```python
from build123d import *

# Parameters (mm, degrees)
F0_R     = 1.25
F1_DEPTH = 7


with BuildPart() as f1:
    # F0 (on Front) → F1 (new body)
    with BuildSketch(Plane.XZ):
        with BuildLine():
            Line((0, 7), (0, 0))
            Line((0, 0), (11, 0))
            Line((11, 0), (11, 7))
            Line((11, 7), (21, 7))
            Line((21, 7), (21, 12))
            Line((21, 12), (20, 12))
            Line((20, 12), (20, 15))
            Line((20, 15), (21, 15))
            Line((21, 15), (21, 21))
            Line((21, 21), (24, 21))
            Line((24, 21), (24, 15))
            Line((24, 15), (25, 15))
            Line((25, 15), (25, 12))
            Line((25, 12), (24, 12))
            Line((24, 12), (24, 7))
            Line((24, 7), (30, 7))
            Line((30, 7), (30, 26))
            Line((30, 26), (0, 26))
            Line((0, 26), (0, 20.75))
            ThreePointArc((0, 20.75), (0.368034, 20.309017), (0.5, 19.75))
            ThreePointArc((0.5, 19.75), (0.368034, 19.190983), (0, 18.75))
            Line((0, 18.75), (0, 7))
        make_face()
        with Locations((8.75, 19.75)):
            Circle(F0_R, mode=Mode.SUBTRACT)
        with BuildLine():
            Line((-5, 7), (0, 7))
            Line((0, 7), (0, 18.75))
            ThreePointArc((0, 18.75), (-2, 19.75), (0, 20.75))
            Line((0, 20.75), (0, 26))
            Line((0, 26), (-5, 26))
            Line((-5, 26), (-5, 7))
        make_face()
    extrude(amount=F1_DEPTH)


solid = f1.part
```
Input: part model. Units: mm. Frame: model coordinates. A direction names the side the tool comes from. Give positions to 0.01 mm unless a question says otherwise; leave off trailing zeros. Order: outer loops, then holes, each group sorted by start corner. A loop starts at its lowest first (then second) coordinate and runs counter-clockwise, first axis right, second up. Notation, with made-up numbers: (84, 82.5) - (101, 82.5) arc R22 ccw to (101, 109.5) - close; hole circle Ø8 at (-9, 66.25). An arc over 180 degrees is marked (long way). One line per item, written item: value.
1. Reachability of faces 1 (the face through (20, -3, 13)), 2 (the face through (5, -3, 0)), 3 (the face through (27, -3, 7)), 4 (the face through (24, -3, 18)), 5 (the face through (0, -3, 4)) from +Z, -Z, +X, -X, +Y, -Y: full face, straight path, thin tool, end or side. Return the list, or none.
Determined:
face 1: +Y, -Y
face 2: -Z, +X, -X, +Y, -Y
face 3: -Z, +X, +Y, -Y
face 4: -Z, +Y, -Y
face 5: -Z, -X, +Y, -Y
2. Draft query along Z for faces 6 (the face through (20.5, -3.5, 12)), 7 (the face through (24, -3, 10)), 8 (the face through (24.5, -3.5, 12)), 9 (the face through (22, -3, 21)). Return one class per face: released by +Z, released by -Z, zero draft, split by the parting line, or undercut.
Determined:
face 6: undercut
face 7: zero draft
face 8: undercut
face 9: released by -Z
3. Cut plane B-B, the plane y = -1. Output: boundary loops of the cut face in (x, z), and give its area (3 significant figures).
Determined:
outline: (-5, 7) - (0, 7) - (0, 0) - (11, 0) - (11, 7) - (21, 7) - (21, 12) - (20, 12) - (20, 15) - (21, 15) - (21, 21) - (24, 21) - (24, 15) - (25, 15) - (25, 12) - (24, 12) - (24, 7) - (30, 7) - (30, 26) - (-5, 26) - close; hole circle Ø2.5 at (-0.75, 19.75); hole circle Ø2.5 at (8.75, 19.75)
area: 684 mm2
4. Pin query (flat end, axial travel): pin 1 Ø3.5 at (y, z) = (-3.5, 2) entering from +X; pin 2 Ø3.5 at (x, y) = (23, -3) entering from -Z; pin 3 Ø2 at (x, z) = (-0.75, 19.75) entering from +Y. Return the tip coordinate at first contact, or that it passes through.
Determined:
pin 1: x = 11
pin 2: z = 7
pin 3: through
5. Line query: probe 1 along X at (y, z) = (-1, 16); probe 2 along Z at (x, y) = (-0.75, -5.25); probe 3 along Z at (x, y) = (8.75, -4.75). Output: solid intervals per line, ascending.
Determined:
probe 1: -5 to 21, 24 to 30
probe 2: 7 to 18.5, 21 to 26
probe 3: 0 to 18.5, 21 to 26
6. Cut plane D-D, the plane z = 19.25. Output: boundary loops of the cut face in (x, y).
Determined:
outline: (-5, -7) - (-1.9, -7) - (-1.9, 0) - (-5, 0) - close; (0.4, -7) - (7.6, -7) - (7.6, 0) - (0.4, 0) - close; (9.9, -7) - (21, -7) - (21, 0) - (9.9, 0) - close; (24, -7) - (30, -7) - (30, 0) - (24, 0) - close
7. Cut plane A-A, the plane z = 8.25. Output: boundary loops of the cut face in (x, y), and give its area (3 significant figures).
Determined:
outline: (-5, -7) - (21, -7) - (21, 0) - (-5, 0) - close; (24, -7) - (30, -7) - (30, 0) - (24, 0) - close
area: 224 mm2
8. Cut plane C-C, the plane x = 8.75. Output: boundary loops of the cut face in (y, z), and give its area (4 significant figures).
Determined:
outline: (-7, 0) - (0, 0) - (0, 18.5) - (-7, 18.5) - close; (-7, 21) - (0, 21) - (0, 26) - (-7, 26) - close
area: 164.5 mm2
